from build123d import *

# Parameters (mm, degrees)
F0_W      = 60.96
F0_H      = 104.14
F1_DEPTH  = 10.414
F2_R      = 5.08
F3_R      = 5.08
F4_R      = 5.08
F5_R      = 5.08
F6_W      = 47.776191
F6_H      = 38.1
F8_DEPTH  = 2.54
F7_R      = 17.78
F7_R_2    = 7.62
F9_DEPTH  = 0.254
F10_R     = 2.403012
F11_DEPTH = 6.35
F12_W     = 24.128942
F12_H     = 2.311272
F13_DEPTH = 5.08


with BuildPart() as f1:
    # F0 (on Top) → F1 (new body)
    with BuildSketch(Plane.XY):
        with Locations((-8.696019, 3.824193)):
            Rectangle(F0_W, F0_H)
    extrude(amount=F1_DEPTH)

    # F2
    f2_edges = [f1.edges().sort_by_distance(p)[0] for p in [
        (21.783981, 55.894193, 5.207),
    ]]
    fillet(f2_edges, radius=F2_R)

    # F3
    f3_edges = [f1.edges().sort_by_distance(p)[0] for p in [
        (-39.176019, 55.894193, 5.207),
    ]]
    fillet(f3_edges, radius=F3_R)

    # F4
    f4_edges = [f1.edges().sort_by_distance(p)[0] for p in [
        (21.783981, -48.245807, 5.207),
    ]]
    fillet(f4_edges, radius=F4_R)

    # F5
    f5_edges = [f1.edges().sort_by_distance(p)[0] for p in [
        (-39.176019, -48.245807, 5.207),
    ]]
    fillet(f5_edges, radius=F5_R)

    # F6 (on face) → F8 (cut)
    with BuildSketch(Plane.XY.offset(10.414)):
        with Locations((-8.627544, 32.658872)):
            Rectangle(F6_W, F6_H)
    extrude(amount=-F8_DEPTH, mode=Mode.SUBTRACT)

    # F7 (on face) → F9 (join)
    with BuildSketch(Plane.XY.offset(10.414)):
        with Locations((-8.950802, -19.304793)):
            Circle(F7_R)
        with Locations((-8.950802, -19.304793)):
            Circle(F7_R_2, mode=Mode.SUBTRACT)
    extrude(amount=F9_DEPTH)

    # F10 (on face) → F11 (cut)
    with BuildSketch(Plane(origin=(0, 55.894193, 0), x_dir=(-1, 0, 0), z_dir=(0, 1, 0))):
        with Locations((-10.893411, 5.443895)):
            Circle(F10_R)
    extrude(amount=-F11_DEPTH, mode=Mode.SUBTRACT)

    # F12 (on face) → F13 (cut)
    with BuildSketch(Plane.XZ.offset(48.245807)):
        with Locations((-8.840048, 5.399611)):
            Rectangle(F12_W, F12_H)
    extrude(amount=-F13_DEPTH, mode=Mode.SUBTRACT)


solid = f1.part
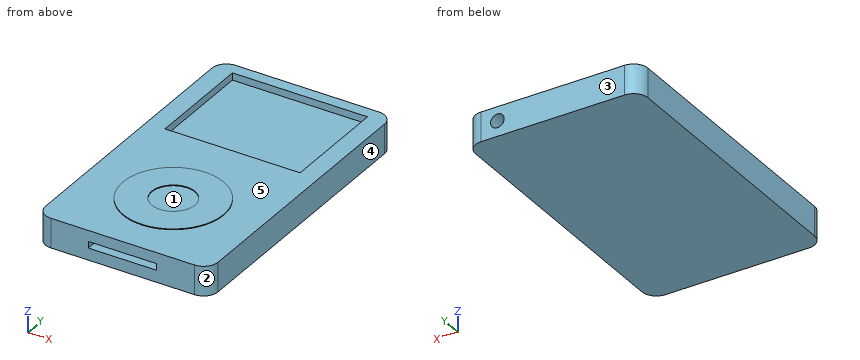
Check sheet for the modelled part. Datum: model origin and axes. Units: mm. Face numbers are marked on the shaded views. A direction names the side the tool comes from. Round coordinates to 2 decimals unless told otherwise and drop trailing zeros. Loops run counter-clockwise (first coordinate to the right, second up) from the corner with the lowest first, then second, coordinate; pieces in that order, holes last. Notation, with made-up numbers: M 75.25,-32.5 L 92.25,-32.5 A14 cw 92.25,-18.5 Z; hole C 6.25,57 d4. An arc over 180 degrees is marked long. One line per question, with ' | ' between items. Start each with the question number.
Item 1: Section check A-A (x = -28). Record the boundary of the cut face in (y, z).
Item 2: Section check B-B (y = 31). Record the boundary of the cut face in (x, z).
Item 3: Release check for a two-part mould opening along X. For the marked faces 1, 2 and 3 record: released by +X, released by -X, zero draft, split by the parting line, or undercut.
Item 4: Scan lines: probe 1 along Y at (x, z) = (0, 10.25); probe 2 along X at (y, z) = (45, 9.75); probe 3 along Z at (x, y) = (-1, 25). Record each from-to range of solid material in increasing order.
Item 5: Set-up check for the marked faces 4 and 5: record each of +Z, -Z, +X, -X, +Y, -Y from which the full face is reachable in a straight line by a thin tool's end or side.
Item 6: Gauge pin test, flat ends, axial feed: pin 1 Ø4 at (x, y) = (-19, -37) entering from +Z; pin 2 Ø1.4 at (x, z) = (12, 4.5) entering from +Y; pin 3 Ø1 at (x, y) = (1, 37.5) entering from +Z. Record the tip position at first contact, or that the pin passes through.
Item 7: Section check C-C (x = -12.5). Record the boundary of the cut face in (y, z).
Item 8: Section check D-D (x = 7.5). Record the boundary of the cut face in (y, z), and give its area (3 significant figures).
Worked out:
1) outline: M -48.25,0 L 55.89,0 L 55.89,10.41 L 51.71,10.41 L 51.71,7.87 L 13.61,7.87 L 13.61,10.41 L -48.25,10.41 Z
2) outline: M -39.18,0 L 21.78,0 L 21.78,10.41 L 15.26,10.41 L 15.26,7.87 L -32.52,7.87 L -32.52,10.41 L -39.18,10.41 Z
3) face 1: undercut | face 2: released by +X | face 3: zero draft
4) probe 1: -48.25 to 13.61, 51.71 to 55.89 | probe 2: -39.18 to -32.52, 15.26 to 21.78 | probe 3: 0 to 7.87
5) face 4: +Z, -Z, +X, +Y, -Y | face 5: +Z
6) pin 1: z = 10.41 | pin 2: y = 49.54 | pin 3: z = 7.87
7) outline: M -48.25,0 L 55.89,0 L 55.89,10.41 L 51.71,10.41 L 51.71,7.87 L 13.61,7.87 L 13.61,10.41 L -1.88,10.41 L -1.88,10.67 L -12.56,10.67 L -12.56,10.41 L -26.05,10.41 L -26.05,10.67 L -36.73,10.67 L -36.73,10.41 L -48.25,10.41 L -48.25,6.56 L -43.17,6.56 L -43.17,4.24 L -48.25,4.24 Z
8) outline: M -48.25,0 L 55.89,0 L 55.89,10.41 L 51.71,10.41 L 51.71,7.87 L 13.61,7.87 L 13.61,10.41 L -12.56,10.41 L -12.56,10.67 L -26.05,10.67 L -26.05,10.41 L -48.25,10.41 Z | area: 991 mm^2
